Design review of the part built by this model. Coordinates are the model's own, in mm. Face numbers are marked on the shaded views. A direction names the side the tool comes from. Coordinates: 2 decimals unless noted, no trailing zeros. Write each loop counter-clockwise with the first axis right and the second up, starting at its lowest first coordinate (ties: lowest second). Pieces come first, ordered by that corner, then holes.
Q1. Machinability: for the marked faces 1 and 2, which of the approach directions +Z, -Z, +X, -X, +Y, -Y give a long, thin tool a straight path to every point of the face, cutting with its end or side? Answer none if there is none.
Q2. Insertion check: pin 1 (0.8 mm diameter, centred on y = 2.5, z = -3, fed in from +X); pin 2 (2 mm diameter, centred on y = 6.5, z = 3, fed in from -X); pin 3 (6 mm diameter, centred on x = 1.5, y = 7, fed in from -Z). Each pin has a flat end and moves straight along its axis. Give the tip position at first contact, or say it passes through.
Q3. Take a section at C-C (x = 10.25). Give the boundary of the cut face in (y, z), and give its area (3 significant figures).
Q4. Take a section at B-B (z = 7.75). Give the boundary of the cut face in (x, y).
Q5. For probe 1 along Z at (x, y) = (-3.5, 6.75); probe 2 along X at (y, z) = (3.25, 1.25); probe 3 along X at (y, z) = (7.5, -7.5), list the stretches that pass through material, from the lowest coordinate up.
Q6. Take a section at D-D (x = -2.75). Give the boundary of the cut face in (y, z), and give its area (3 significant figures).
Q7. Mouldability with a two-part tool opening along Z and no side actions: class the marked faces 3, 4 and 5 as pulls with the +Z half, pulls with the -Z half, needs draft (parallel to the pull), parting line crosses it, or undercut.
Autodesk Inventor part; units mm, degrees
ref_plane "YZ Plane" through (0, 0, 0) normal (1, 0, 0) x (0, 1, 0)
ref_plane "XZ Plane" through (0, 0, 0) normal (0, 1, 0) x (-1, 0, 0)
ref_plane "XY Plane" through (0, 0, 0) normal (0, 0, 1) x (1, 0, 0)
sketch "Sketch1" plane through (0, 0, 0) normal (0, 1, 0) x (-1, 0, 0)
  line L0 (-10, 10) -> (10, 10)
  line L1 (10, 10) -> (10, -10)
  line L2 (10, -10) -> (-10, -10)
  line L3 (-10, -10) -> (-10, 10)
  line L4 (-10, 10) -> (10, -10) construction
  line L5 (10, 10) -> (-10, -10) construction
  line L6 (-9.5, 0) -> (-4.75, 8.2272)
  line L7 (-4.75, 8.2272) -> (4.75, 8.2272)
  line L8 (4.75, 8.2272) -> (9.5, 0)
  line L9 (9.5, 0) -> (4.75, -8.2272)
  line L10 (4.75, -8.2272) -> (-4.75, -8.2272)
  line L11 (-4.75, -8.2272) -> (-9.5, 0)
  line L12 (-8.3453, 0) -> (-4.1726, 7.2272)
  line L13 (-4.1726, 7.2272) -> (4.1726, 7.2272)
  line L14 (4.1726, 7.2272) -> (8.3453, 0)
  line L15 (8.3453, 0) -> (4.1726, -7.2272)
  line L16 (4.1726, -7.2272) -> (-4.1726, -7.2272)
  line L17 (-4.1726, -7.2272) -> (-8.3453, 0)
  line L18 (2.1284, -3.7272) -> (2.1284, -2.2272)
  line L19 (2.1284, -2.2272) -> (3.6284, -2.2272)
  line L20 (3.6284, -2.2272) -> (3.6284, -4.7272)
  line L21 (3.6284, -4.7272) -> (0, -4.7272)
  line L22 (0, -4.7272) -> (0, -2.2272)
  line L23 (0, -2.2272) -> (0.7279, -0.2272)
  line L24 (0.7279, -0.2272) -> (0, -0.2272)
  line L25 (0, -0.2272) -> (0, 0.7728)
  line L26 (0, 0.7728) -> (1.0919, 0.7728)
  line L27 (3.2314, 3.7272) -> (0.5182, -3.7272)
  line L28 (0.5182, -3.7272) -> (2.1284, -3.7272)
  line L29 (3.2314, 3.7272) -> (4.116, 3.7272)
  line L30 (4.116, 3.7272) -> (4.116, 2.2272)
  line L31 (4.116, 2.2272) -> (5.616, 2.2272)
  line L32 (5.616, 2.2272) -> (5.616, 4.7272)
  line L33 (5.616, 4.7272) -> (2.2598, 4.7272)
  line L34 (1.0919, 0.7728) -> (2.1673, 3.7272)
  line L35 (2.1673, 3.7272) -> (0.5571, 3.7272)
  line L36 (0.5571, 3.7272) -> (0.5571, 2.2272)
  line L37 (0.5571, 2.2272) -> (0, 2.2272)
  line L38 (0, 2.2272) -> (0, 4.7272)
  line L39 (0, 4.7272) -> (2.2598, 4.7272)
  line L40 (-2.1284, -3.7272) -> (-2.1284, -2.2272)
  line L41 (-2.1284, -2.2272) -> (-3.6284, -2.2272)
  line L42 (-3.6284, -2.2272) -> (-3.6284, -4.7272)
  line L43 (-3.6284, -4.7272) -> (0, -4.7272)
  line L44 (0, -2.2272) -> (-0.7279, -0.2272)
  line L45 (-0.7279, -0.2272) -> (0, -0.2272)
  line L46 (0, 0.7728) -> (-1.0919, 0.7728)
  line L47 (-3.2314, 3.7272) -> (-0.5182, -3.7272)
  line L48 (-0.5182, -3.7272) -> (-2.1284, -3.7272)
  line L49 (-3.2314, 3.7272) -> (-4.116, 3.7272)
  line L50 (-4.116, 3.7272) -> (-4.116, 2.2272)
  line L51 (-4.116, 2.2272) -> (-5.616, 2.2272)
  line L52 (-5.616, 2.2272) -> (-5.616, 4.7272)
  line L53 (-5.616, 4.7272) -> (-2.2598, 4.7272)
  line L54 (-1.0919, 0.7728) -> (-2.1673, 3.7272)
  line L55 (-2.1673, 3.7272) -> (-0.5571, 3.7272)
  line L56 (-0.5571, 3.7272) -> (-0.5571, 2.2272)
  line L57 (-0.5571, 2.2272) -> (0, 2.2272)
  line L58 (0, 4.7272) -> (-2.2598, 4.7272)
  line L59 (5.616, -8.7272) -> (9.5, -2)
  line L60 (9.5, -2) -> (9.5, -9.7272)
  line L61 (9.5, -9.7272) -> (0, -9.7272)
  line L62 (0, -9.7272) -> (0, -8.7272)
  line L63 (0, -8.7272) -> (5.616, -8.7272)
  line L64 (6.7707, -8.7272) -> (8.5, -8.7272)
  line L65 (8.5, -8.7272) -> (8.5, -5.7321)
  line L66 (8.5, -5.7321) -> (6.7707, -8.7272)
  line L67 (-5.616, -8.7272) -> (-9.5, -2)
  line L68 (-9.5, -2) -> (-9.5, -9.7272)
  line L69 (-9.5, -9.7272) -> (0, -9.7272)
  line L70 (0, -8.7272) -> (-5.616, -8.7272)
  line L71 (-6.7707, -8.7272) -> (-8.5, -8.7272)
  line L72 (-8.5, -8.7272) -> (-8.5, -5.7321)
  line L73 (-8.5, -5.7321) -> (-6.7707, -8.7272)
  line L74 (10, 0) -> (14.2645, 0) construction
  line L75 (-10, -10) -> (10, 10) construction
  line L76 (4.75, 8.2272) -> (-4.75, 8.2272)
  line L77 (5.616, 8.7272) -> (9.5, 2)
  line L78 (9.5, 2) -> (9.5, 9.7272)
  line L79 (9.5, 9.7272) -> (0, 9.7272)
  line L80 (0, 9.7272) -> (0, 8.7272)
  line L81 (0, 8.7272) -> (5.616, 8.7272)
  line L82 (6.7707, 8.7272) -> (8.5, 8.7272)
  line L83 (8.5, 8.7272) -> (8.5, 5.7321)
  line L84 (8.5, 5.7321) -> (6.7707, 8.7272)
  line L85 (-9.5, 9.7272) -> (0, 9.7272)
  line L86 (-6.7707, 8.7272) -> (-8.5, 8.7272)
  line L87 (-8.5, 5.7321) -> (-6.7707, 8.7272)
  line L88 (-8.5, 8.7272) -> (-8.5, 5.7321)
  line L89 (-9.5, 2) -> (-9.5, 9.7272)
  line L90 (-5.616, 8.7272) -> (-9.5, 2)
  line L91 (0, 8.7272) -> (-5.616, 8.7272)
  point P0 (0, 0)
  point P1 (0, 0)
  point P2 (0, 0)
  point P3 (0, -7.2272)
  dimension "d0" = 20
  dimension "d1" = 20
  dimension "d2" = 0.5
  dimension "d3" = 1
  dimension "d4" = 1.5
  dimension "d5" = 1
  dimension "d6" = 1.5
  dimension "d7" = 1
  dimension "d9" = 70
  dimension "d13" = 1.5
  dimension "d14" = 1.5
  dimension "d15" = 1
  dimension "d16" = 1
  dimension "d17" = 2
  dimension "d18" = 1
  dimension "d19" = 2.5
  dimension "d23" = 1
  dimension "d26" = 2.5
  dimension "d29" = 0.5
  dimension "d30" = 1
  dimension "d32" = 1
  dimension "d33" = 1
  dimension "d34" = 1
extrude "Extrusion1" add sketch "Sketch1" along normal blind 10 contours L6 L7 L8 L9 L10 L11 | L53 L58 L38 L57 L56 L55 L54 L46 L25 L45 L44 L22 L43 L42 L41 L40 L48 L47 L49 L50 L51 L52 | L39 L33 L32 L31 L30 L29 L27 L28 L18 L19 L20 L21 L22 L23 L24 L25 L26 L34 L35 L36 L37 L38 | L59 L60 L61 L62 L63 | L62 L69 L68 L67 L70 | L81 L80 L79 L78 L77 | L91 L90 L89 L85 L80
sketch "Sketch2" plane through (0, 0, 0) normal (0, 1, 0) x (-1, 0, 0)
  line L0 (-15, 15) -> (15, 15)
  line L1 (15, 15) -> (15, -15)
  line L2 (15, -15) -> (-15, -15)
  line L3 (-15, -15) -> (-15, 15)
  line L4 (-15, 15) -> (15, -15) construction
  line L5 (15, 15) -> (-15, -15) construction
  point P0 (0, 0)
  dimension "d35" = 30
  dimension "d36" = 30
extrude "Extrusion2" add sketch "Sketch2" against normal blind 0.2
equation "\"d2\" = mini"
equation "\"d3\" = 2 * mini"
equation "\"nozzleHead\" = 0.5"
equation "\"mini\" = nozzleHead"
properties part number "A_main"
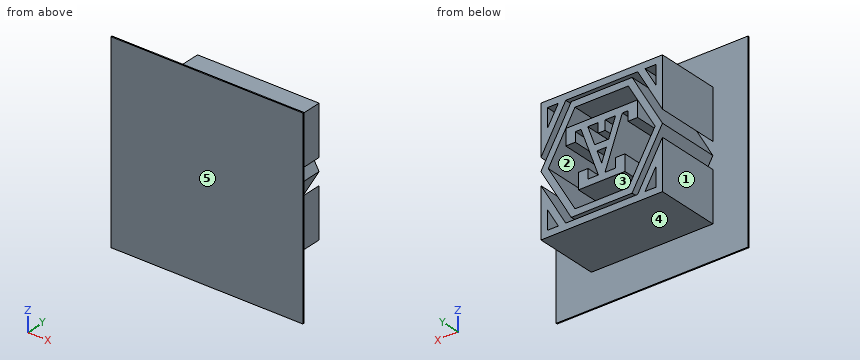
Response:
1. face 1: +Z, -Z, -X, +Y
1. face 2: +Y
2. pin 1: stops at x = 9.5
2. pin 2: stops at x = -9.5
2. pin 3: stops at z = -9.73
3. outline: (-0.2, -15) - (0, -15) - (0, 15) - (-0.2, 15) - close
3. area: 6.00 mm2
4. outline: (-15, -0.2) - (15, -0.2) - (15, 0) - (9.5, 0) - (9.5, 10) - (8.5, 10) - (8.5, 0) - (7.33, 0) - (7.33, 10) - (6.18, 10) - (6.18, 0) - (5.03, 0) - (5.03, 10) - (-5.03, 10) - (-5.03, 0) - (-6.18, 0) - (-6.18, 10) - (-7.33, 10) - (-7.33, 0) - (-8.5, 0) - (-8.5, 10) - (-9.5, 10) - (-9.5, 0) - (-15, 0) - close
5. probe 1: z = -9.73 to -8.73, -8.23 to -7.23, -4.73 to -2.23, 3.73 to 4.73, 7.23 to 8.23, 8.73 to 9.73
5. probe 2: x = -8.78 to -7.62, -2.33 to -1.27, 1.27 to 2.33, 7.62 to 8.78
5. probe 3: x = -9.5 to -8.5, -7.48 to -6.32, -5.17 to 5.17, 6.32 to 7.48, 8.5 to 9.5
6. outline: (-0.2, -15) - (0, -15) - (0, -9.73) - (10, -9.73) - (10, -8.73) - (0, -8.73) - (0, -8.23) - (10, -8.23) - (10, -7.23) - (0, -7.23) - (0, -4.73) - (10, -4.73) - (10, -2.23) - (0, -2.23) - (0, 2.4) - (10, 2.4) - (10, 4.73) - (0, 4.73) - (0, 7.23) - (10, 7.23) - (10, 8.23) - (0, 8.23) - (0, 8.73) - (10, 8.73) - (10, 9.73) - (0, 9.73) - (0, 15) - (-0.2, 15) - close
6. area: 94.2 mm2
7. face 3: undercut
7. face 4: pulls with the -Z half
7. face 5: needs draft
